Verification items for this drawing (mm, ordinates from the low corner). Round coordinates to 2 decimals unless told otherwise and drop trailing zeros. Write each loop counter-clockwise with the first axis right and the second up, starting at its lowest first coordinate (ties: lowest second). Pieces come first, ordered by that corner, then holes. Notation, with made-up numbers: (-2.5, 62.5) -> (42.5, 62.5) arc R6 cw to (42.5, 68.5) -> close; hole circle Ø4 at (67, 85.5). An arc over 180 degrees is marked (long way). Return JSON: item names as keys, results as strings. Group by question number.
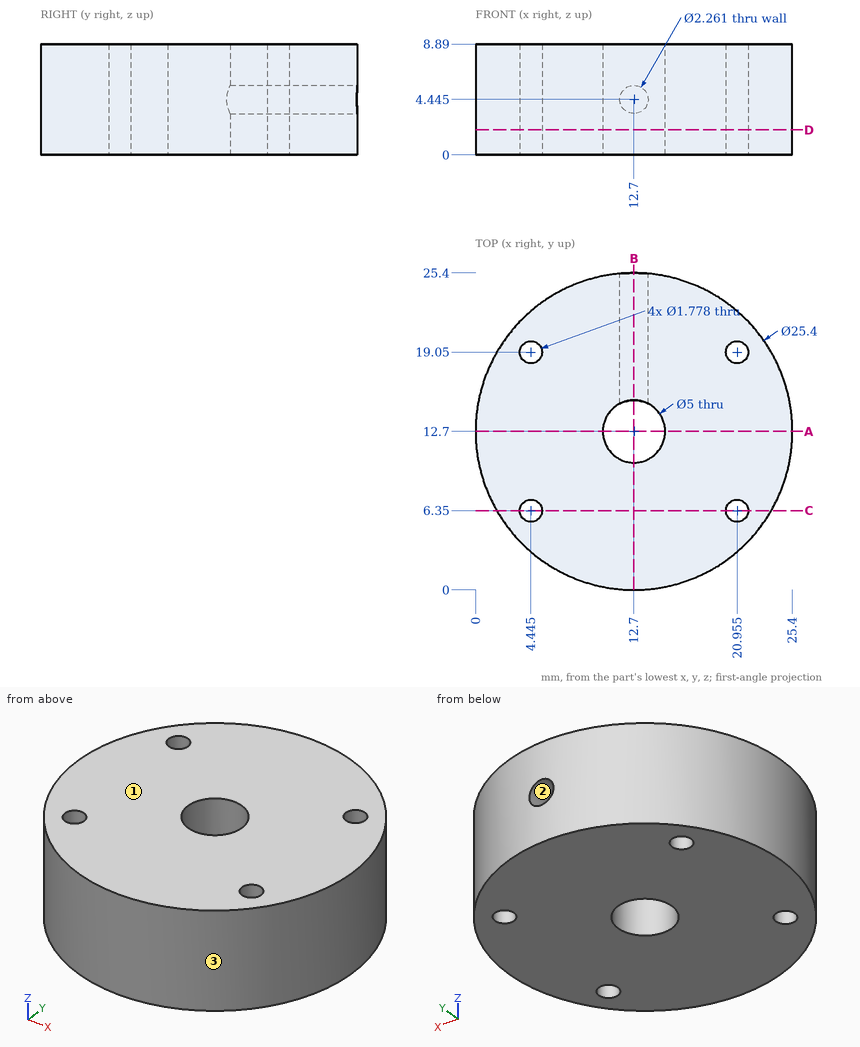
1) Sectioned sample at A-A on y = 12.7. Enter the section's corners in (x, z).
2) Go/stop test with flat-tipped pins: P1, Ø1.5, axis at y = 21, z = 6.5, coming from the +X side; P2, Ø1.4, axis at x = 4.445, y = 19.05, coming from the -Z side; P3, Ø2, axis at x = 5.5, z = 3.5, coming from the +Y side. Record where each tip stops, or that it passes through.
3) Material ranges on probe 1 along X at (y, z) = (14.5, 7.25) (1 decimal); probe 2 along Y at (x, z) = (13.75, 2) (1 decimal); probe 3 along Z at (x, y) = (11.75, 15.5) (1 decimal), recorded low to high. Write a range as [from, to].
4) Sectioned sample at C-C on y = 6.35. Enter the section's corners in (x, z), and give its area (3 significant figures).
5) Sectioned sample at B-B on x = 12.7. Enter the section's corners in (y, z) (1 decimal).
6) Sectioned sample at D-D on z = 2. State how many separate pieces and enclosed holes the cut face has, and give its area (3 significant figures).
7) Mould release check, pull along X, two halves, no side actions. Record for the marked faces 1, 2 and 3: +X half, -X half, draft (parallel to the pull), parting line (faces both ways), or undercut.
Evaluation:
{
 "1": {"outline": "(0, 0) -> (10.2, 0) -> (10.2, 8.89) -> (0, 8.89) -> close; (15.2, 0) -> (25.4, 0) -> (25.4, 8.89) -> (15.2, 8.89) -> close"},
 "2": {"P1": "stops at x = 22.91", "P2": "passes through", "P3": "stops at y = 23.78"},
 "3": {"probe 1": "x = [0.1, 11], [14.4, 25.3]", "probe 2": "y = [0, 10.4], [15, 25.4]", "probe 3": "z = [0, 3.8], [5.1, 8.9]"},
 "4": {"outline": "(1.7, 0) -> (3.56, 0) -> (3.56, 8.89) -> (1.7, 8.89) -> close; (5.33, 0) -> (20.07, 0) -> (20.07, 8.89) -> (5.33, 8.89) -> close; (21.84, 0) -> (23.7, 0) -> (23.7, 8.89) -> (21.84, 8.89) -> close", "area": "164 mm2"},
 "5": {"outline": "(0, 0) -> (10.2, 0) -> (10.2, 8.9) -> (0, 8.9) -> close; (15.2, 0) -> (25.4, 0) -> (25.4, 3.3) -> (15.2, 3.3) -> close; (15.2, 5.6) -> (25.4, 5.6) -> (25.4, 8.9) -> (15.2, 8.9) -> close"},
 "6": {"separate pieces": "1", "enclosed holes": "5", "area": "477 mm2"},
 "7": {"face 1": "draft", "face 2": "undercut", "face 3": "parting line"}
}
